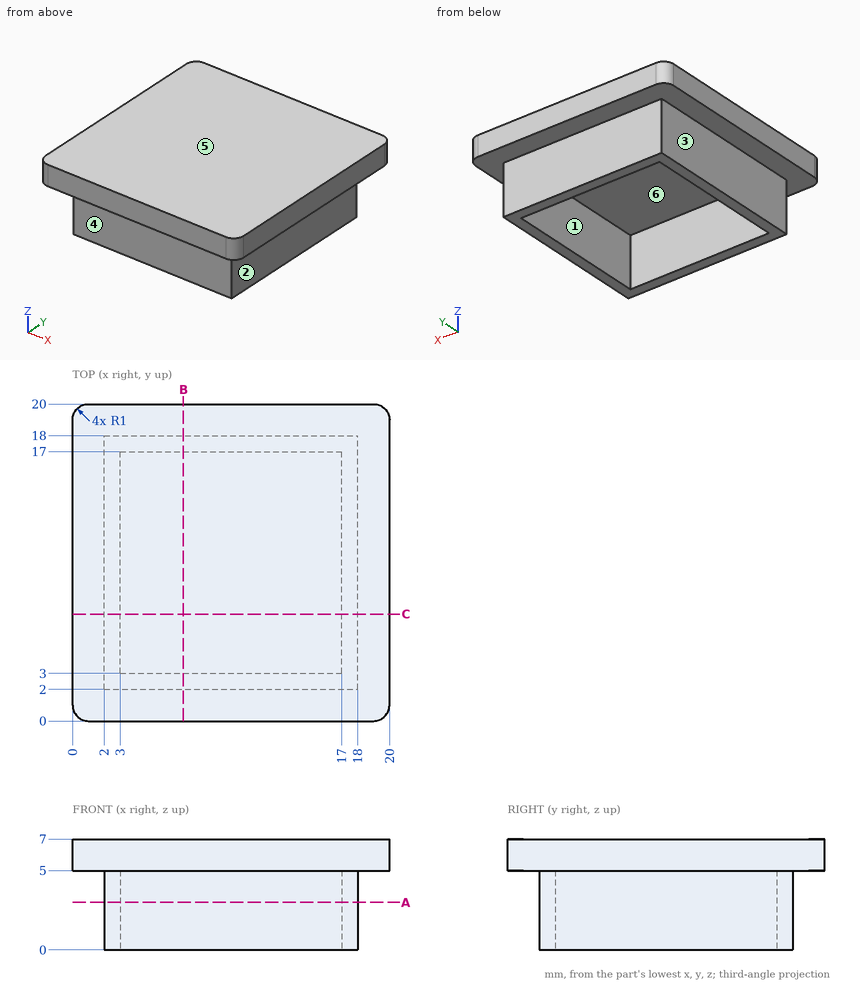
Geometry: see drawing. Coordinates: mm, zero at the bounding-box minimum. A direction names the side the tool comes from. Round coordinates to 2 decimals unless told otherwise and drop trailing zeros. Order: outer loops, then holes, each group sorted by start corner. A loop starts at its lowest first (then second) coordinate and runs counter-clockwise, first axis right, second up. Notation, with made-up numbers: (2.5, 38) - (45.5, 38) arc R25 ccw to (45.5, 53) - close; hole circle Ø5 at (-36, -17). An arc over 180 degrees is marked (long way). One line per question, with ' | ' between items. Start each with the question number.
1) Contact query for flat-ended pins moving along their axis: P1, Ø1.5, axis at y = 7.5, z = 2, coming from the -X side; P2, Ø2.5, axis at x = 9.5, z = 3.5, coming from the -Y side; P3, Ø2.5, axis at y = 14, z = 3.5, coming from the +X side. Output: stop coordinate, or through.
2) Set-up query: the marked faces 1, 2 and 3. Return all of +Z, -Z, +X, -X, +Y, -Y with unobstructed straight access to the full face (end or side cutting, diameter ignored); none if empty.
3) Cut plane B-B, the plane x = 7. Return the cut outline in (y, z), then the cut area to 3 significant figures.
4) Cut plane A-A, the plane z = 3. Return the cut outline in (x, y).
5) Ray query, probe 1 along Y at (x, z) = (4, 0.5); probe 2 along Z at (x, y) = (12.25, 18.75). Return the intervals inside material, ascending.
6) Pull-direction query (Y, two-part tool) for the marked faces 4, 5 and 6; classes: +Y half, -Y half, draft (parallel to the pull), parting line (faces both ways), or undercut.
Worked out:
1) P1: stops at x = 2 | P2: stops at y = 2 | P3: stops at x = 18
2) face 1: -Z | face 2: -Z, +X, +Y, -Y | face 3: -Z, -X, +Y, -Y
3) outline: (0, 5) - (2, 5) - (2, 0) - (3, 0) - (3, 5) - (17, 5) - (17, 0) - (18, 0) - (18, 5) - (20, 5) - (20, 7) - (0, 7) - close | area: 50.0 mm^2
4) outline: (2, 2) - (18, 2) - (18, 18) - (2, 18) - close; hole (3, 3) - (17, 3) - (17, 17) - (3, 17) - close
5) probe 1: y = 2 to 3, 17 to 18 | probe 2: z = 5 to 7
6) face 4: -Y half | face 5: draft | face 6: undercut
